For this review, take the finished solid that the model builds, in its own axes (mm). Give positions to 0.01 mm unless a question says otherwise; leave off trailing zeros. Loops run counter-clockwise (first coordinate to the right, second up) from the corner with the lowest first, then second, coordinate; pieces in that order, holes last. Notation, with made-up numbers: (56.5, 57) - (108.5, 57) arc R27 cw to (108.5, 85) - close; hole circle Ø5 at (41.25, 9.5). An arc over 180 degrees is marked (long way). Put each result on its own line as item: value.
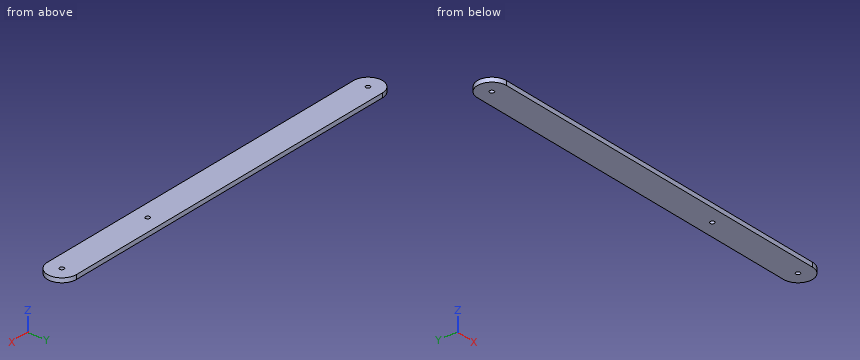
Autodesk Inventor part; units mm, degrees
ref_plane "YZ Plane" through (0, 0, 0) normal (1, 0, 0) x (0, 1, 0)
ref_plane "XZ Plane" through (0, 0, 0) normal (0, 1, 0) x (-1, 0, 0)
ref_plane "XY Plane" through (0, 0, 0) normal (0, 0, 1) x (1, 0, 0)
sketch "Skizze1" plane through (0, 0, 0) normal (0, 0, 1) x (1, 0, 0)
  line L0 (-189.879, 0) -> (188.121, 0)
  line L1 (0, -8.5091) -> (0, 51.0549)
  line L2 (-125.879, 42.5457) -> (124.121, 42.5457)
  line L3 (124.121, 22.5457) -> (-125.879, 22.5457)
  arc A0 (-125.879, 42.5457) -> (-125.879, 22.5457) centre (-125.879, 32.5457) ccw
  arc A1 (124.121, 22.5457) -> (124.121, 42.5457) centre (124.121, 32.5457) ccw
  point P0 (0, 0)
  dimension "d5" = 250
  dimension "d6" = 20
extrude "Extrusion1" add sketch "Skizze1" along normal blind 3
sketch "Skizze2" plane through (0, 0, 3) normal (0, 0, 1) x (1, 0, 0)
  arc A0 (124.121, 22.5457) -> (124.121, 42.5457) centre (124.121, 32.5457) ccw
  line L0 (124.121, 42.5457) -> (-125.879, 42.5457)
  arc A1 (-125.879, 42.5457) -> (-125.879, 22.5457) centre (-125.879, 32.5457) ccw
  point P0 (0, 0)
  point P1 (-125.879, 32.5457)
  dimension "d9" = 10
  dimension "d10" = 0
hole "Bohrung1" at (-125.879, 32.5457, 3) at (124.121, 32.5457, 3) direction (0, 0, -1) diameter 3 depth 57.1 tip angle 118
sketch "Skizze3" plane through (0, 0, 3) normal (0, 0, 1) x (1, 0, 0)
  circle A0 centre (124.121, 32.5457) radius 1.5
  line L0 (124.121, 42.5457) -> (-125.879, 42.5457)
  point P0 (0, 0)
  point P1 (54.121, 32.5457)
  dimension "d18" = 70
  dimension "d19" = 10
hole "Bohrung2" at (54.121, 32.5457, 3) direction (0, 0, -1) diameter 3 depth 57.1 tip angle 118
properties part number "Träger vorne oben lang"
1) Take a section at A-A on z = 0.8. State the section outline as (x, y) points.
Geometry check:
outline: (-125.88, 22.55) - (124.12, 22.55) arc R10 ccw to (124.12, 42.55) - (-125.88, 42.55) arc R10 ccw to start; hole circle Ø3 at (-125.88, 32.55); hole circle Ø3 at (54.12, 32.55); hole circle Ø3 at (124.12, 32.55)
2) Insertion check: pin 1 Ø2.5 at (x, y) = (-125.88, 32.55) entering from -Z. The pin has a flat end and moves straight along its axis. Give the tip position at first contact, or say it passes through.
Geometry check:
pin 1: passes through
3) Take a section at B-B on y = 39.75. State the section outline as (x, z) points, and give its area (3 significant figures).
Geometry check:
outline: (-132.81, 0) - (131.06, 0) - (131.06, 3) - (-132.81, 3) - close
area: 792 mm²
4) Wall thickness on line 1 (X direction, y = 32.75, z = 0.2); line 2 (X direction, y = 31.5, z = 1.5); line 3 (X direction, y = 29.25, z = 2.85): over which ranges is each line inside the solid? List them lowest first.
Geometry check:
line 1: x = -135.88 to -127.37, -124.39 to 52.63, 55.61 to 122.63, 125.61 to 134.12
line 2: x = -135.82 to -126.95, -124.8 to 53.05, 55.2 to 123.05, 125.2 to 134.07
line 3: x = -135.32 to 133.56
